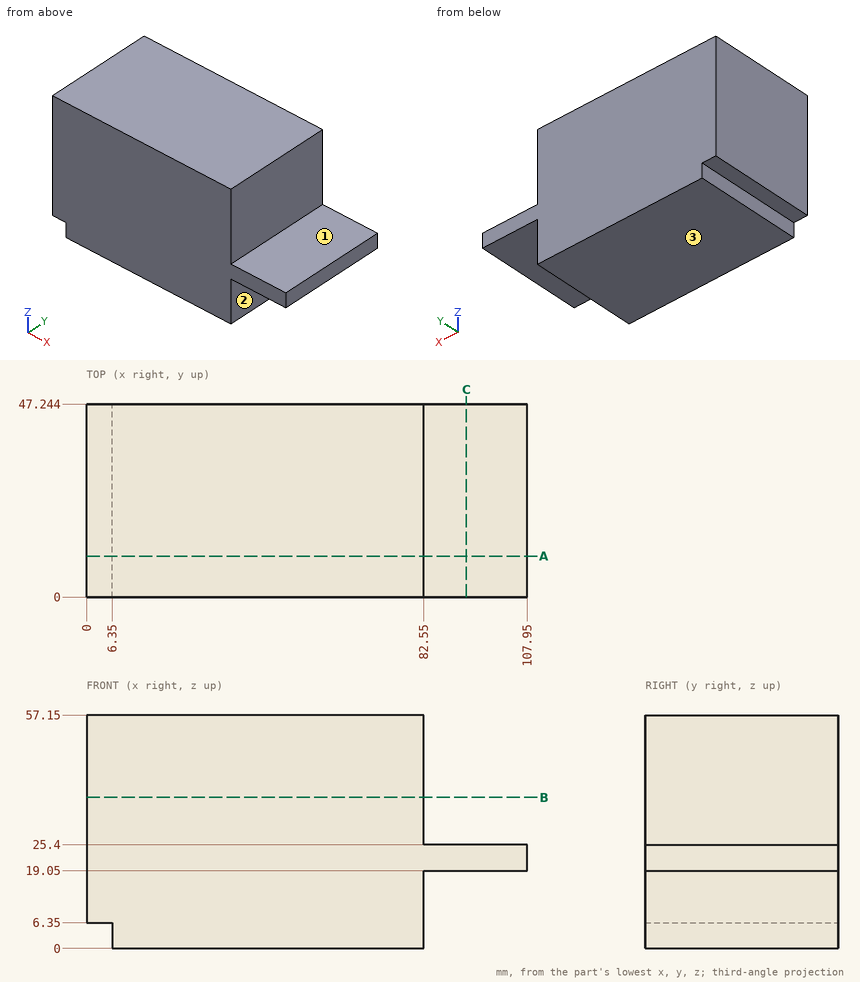
The drawing under review shows one solid part. Ordinate dimensions are in mm from its lowest x, y, z. A direction names the side the tool comes from. Coordinates: 2 decimals unless noted, no trailing zeros. Order: outer loops, then holes, each group sorted by start corner. A loop starts at its lowest first (then second) coordinate and runs counter-clockwise, first axis right, second up. Notation, with made-up numbers: (87, 16.25) -> (137, 16.25) arc R22 ccw to (137, 41.25) -> close; hole circle Ø10 at (85, -20). An arc over 180 degrees is marked (long way). Return JSON: item names as keys, results as strings.
1. We need section C-C on x = 93. Write out the cut boundary in (y, z), and give its area (3 significant figures).
Answer block:
{"outline": "(0, 19.05) -> (47.24, 19.05) -> (47.24, 25.4) -> (0, 25.4) -> close", "area": "300 mm²"}
2. For line 1 (Z direction, x = 93.5, y = 6.5); line 2 (X direction, y = 34, z = 50), list the stretches that pass through material, from the lowest coordinate up. Write a range as from..to.
Answer block:
{"line 1": "19.05..25.4", "line 2": "0..82.55"}
3. We need section B-B on z = 37. Write out the cut boundary in (x, y), and give its area (3 significant figures).
Answer block:
{"outline": "(0, 0) -> (82.55, 0) -> (82.55, 47.24) -> (0, 47.24) -> close", "area": "3,900 mm²"}
4. Machinability: for the marked faces 1, 2 and 3, which of the approach directions +Z, -Z, +X, -X, +Y, -Y give a long, thin tool a straight path to every point of the face, cutting with its end or side? Answer none if there is none.
Answer block:
{"face 1": "+Z, +X, +Y, -Y", "face 2": "-Z, +X, +Y, -Y", "face 3": "-Z, +X, -X, +Y, -Y"}
5. For pin 1 Ø9.5 at (y, z) = (12.5, 34) entering from +X; pin 2 Ø3 at (x, y) = (3, 30) entering from -Z; pin 3 Ø5 at (x, y) = (87.5, 6.5) entering from -Z, all flat-tipped, find the tip position at first contact; note any pin that passes through.
Answer block:
{"pin 1": "x = 82.55", "pin 2": "z = 6.35", "pin 3": "z = 19.05"}
6. We need section A-A on y = 10. Write out the cut boundary in (x, z), and give its area (3 significant figures).
Answer block:
{"outline": "(0, 6.35) -> (6.35, 6.35) -> (6.35, 0) -> (82.55, 0) -> (82.55, 19.05) -> (107.95, 19.05) -> (107.95, 25.4) -> (82.55, 25.4) -> (82.55, 57.15) -> (0, 57.15) -> close", "area": "4,840 mm²"}
